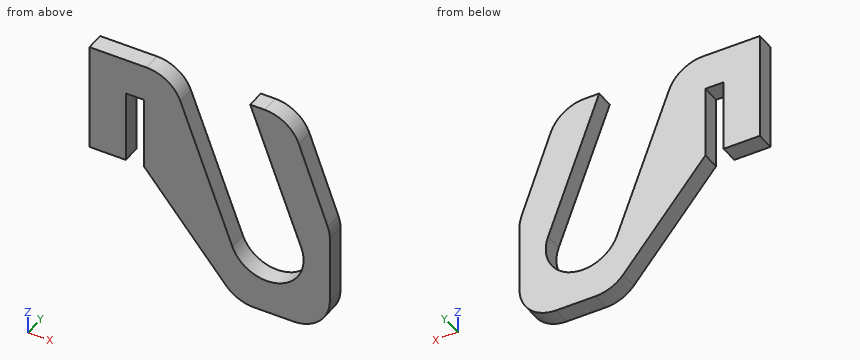
from build123d import *

# Parameters (mm, degrees)
F1_DEPTH = 3.175


# Not quite as in the source:
# - a length typed as a fraction of an inch, garbled in the dataset ("3 / 203.2 mm" for 3/8 in), is restored


with BuildPart() as f1:
    # F0 (on Front) → F1 (new body)
    with BuildSketch(Plane.XZ):
        with BuildLine():
            Line((0, 19.05), (0, 0))
            Line((0, 0), (6.35, 0))
            Line((6.35, 0), (6.35, 12.7))
            Line((6.35, 12.7), (9.525, 12.7))
            Line((9.525, 12.7), (9.525, 0))
            Line((9.525, 0), (23.8846407704, -17.1268223527))
            ThreePointArc((23.8846407704, -17.1268223527), (26.0658700781, -18.8015604613), (28.7506271903, -19.3970336129))
            Line((28.7506271903, -19.3970336129), (35.7011077573, -19.3970336129))
            ThreePointArc((35.7011077573, -19.3970336129), (40.1912358178, -17.5371616734), (42.0511077573, -13.0470336129))
            Line((42.0511077573, -13.0470336129), (42.0511077573, -1.1253461624))
            ThreePointArc((42.0511077573, -1.1253461624), (41.9536799226, -0.017266148), (41.6643860823, 1.0568113981))
            Line((41.6643860823, 1.0568113981), (36.6052420996, 14.8821575605))
            ThreePointArc((36.6052420996, 14.8821575605), (34.2796690603, 17.9047670702), (30.6419637747, 19.05))
            Line((30.6419637747, 19.05), (28.1090781347, 19.05))
            Line((28.1090781347, 19.05), (37.0488404527, -4.7744145618))
            ThreePointArc((37.0488404527, -4.7744145618), (33.2823465228, -13.0652413354), (24.9915197492, -9.2987474054))
            Line((24.9915197492, -9.2987474054), (15.8997145825, 14.9308604634))
            ThreePointArc((15.8997145825, 14.9308604634), (13.5708732383, 17.9196007483), (9.9544844278, 19.05))
            Line((9.9544844278, 19.05), (0, 19.05))
        make_face()
    extrude(amount=F1_DEPTH)


solid = f1.part
The model under review builds one solid part; all positions refer to its coordinate system, in mm. Round coordinates to 2 decimals unless told otherwise and drop trailing zeros. Write each loop counter-clockwise with the first axis right and the second up, starting at its lowest first coordinate (ties: lowest second). Pieces come first, ordered by that corner, then holes. Notation, with made-up numbers: (53, 37.5) -> (106, 37.5) arc R8 cw to (106, 45.5) -> close; hole circle Ø7 at (73.25, 68.25). An arc over 180 degrees is marked (long way). Answer as a JSON object with one key per item and string values.
1. We need section A-A on z = 2.5. State the section outline as (x, y) points (3 decimals), and give its area (3 significant figures).
Results found:
{"outline": "(0, -3.175) -> (6.35, -3.175) -> (6.35, 0) -> (0, 0) -> close; (9.525, -3.175) -> (20.564, -3.175) -> (20.564, 0) -> (9.525, 0) -> close; (34.319, -3.175) -> (41.136, -3.175) -> (41.136, 0) -> (34.319, 0) -> close", "area": "76.9 mm^2"}
2. To check wall thickness, follow line 1 along X through (y, z) = (-0.85, 16); line 2 along X through (y, z) = (-0.4, -13); line 3 along X through (y, z) = (-0.5, 12) (3 decimals). State the ranges of each line that lie inside material, in increasing order.
Results found:
{"line 1": "x = 0 to 15.38, 29.25 to 36.07", "line 2": "x = 20.42 to 28.59, 33.45 to 42.05", "line 3": "x = 0 to 6.35, 9.525 to 16.999, 30.754 to 37.66"}
3. Clearance check with flat-ended pins moving along their axes: pin 1 (1 mm diameter, centred on x = 1.5, y = -1.5, fed in from -Z); pin 2 (1 mm diameter, centred on x = 7, y = -1.5, fed in from -Z). State where each tip first meets the part, or that it passes through.
Results found:
{"pin 1": "stops at z = 0", "pin 2": "stops at z = 12.7"}
4. We need section B-B on y = -2.5. State the section outline as (x, z) points (3 decimals), and give its area (3 significant figures).
Results found:
{"outline": "(0, 0) -> (6.35, 0) -> (6.35, 12.7) -> (9.525, 12.7) -> (9.525, 0) -> (23.885, -17.127) arc R6.35 ccw to (28.751, -19.397) -> (35.701, -19.397) arc R6.35 ccw to (42.051, -13.047) -> (42.051, -1.125) arc R6.35 ccw to (41.664, 1.057) -> (36.605, 14.882) arc R6.35 ccw to (30.642, 19.05) -> (28.109, 19.05) -> (37.049, -4.774) arc R6.439 cw to (24.992, -9.299) -> (15.9, 14.931) arc R6.35 ccw to (9.954, 19.05) -> (0, 19.05) -> close", "area": "727 mm^2"}
5. We need section D-D on z = -3. State the section outline as (x, y) points (3 decimals), and give its area (3 significant figures).
Results found:
{"outline": "(12.04, -3.175) -> (22.628, -3.175) -> (22.628, 0) -> (12.04, 0) -> close; (36.383, -3.175) -> (42.051, -3.175) -> (42.051, 0) -> (36.383, 0) -> close", "area": "51.6 mm^2"}
6. We need section C-C on x = 30. State the section outline as (y, z) points (3 decimals), and give its area (3 significant figures).
Results found:
{"outline": "(-3.175, -19.397) -> (0, -19.397) -> (0, -13.394) -> (-3.175, -13.394) -> close; (-3.175, 14.011) -> (0, 14.011) -> (0, 19.05) -> (-3.175, 19.05) -> close", "area": "35.1 mm^2"}
